CAD build for the part. Positions are in the model's coordinates, mm. A direction names the side the tool comes from. Round coordinates to 2 decimals unless told otherwise and drop trailing zeros. Loops run counter-clockwise (first coordinate to the right, second up) from the corner with the lowest first, then second, coordinate; pieces in that order, holes last.
from build123d import *

# Parameters (mm, degrees)
CUT_EXTRUDE_1_DEPTH = 4
CUT_EXTRUDE_2_DEPTH = 5


with BuildPart() as part:
    # 草图1 → 旋转1 (revolve)
    with BuildSketch(Plane(origin=(0, 0, 0), x_dir=(1, 0, 0), z_dir=(0, 1, 0)), mode=Mode.PRIVATE) as revolve_1_sk:
        Polygon((-128.123292873, 0), (-128.123292873, 15.5), (-126.123292873, 17.5), (-96.123292873, 17.5), (-96.123292873, 21), (-88.123292873, 21), (-88.123292873, 19), (-36.123292873, 19), (-36.123292873, 17.5), (5.876707127, 17.5), (5.876707127, 15), (48.876707127, 15), (48.876707127, 12.5), (106.876707127, 12.5), (108.876707127, 10.5), (108.876707127, 0), align=None)
    revolve(revolve_1_sk.sketch.rotate(Axis((-128.123292873, 0, 0), (1, 0, 0)), 180), axis=Axis((-128.123292873, 0, 0), (1, 0, 0)))

    # 草图2 → 切除-拉伸1 (cut)
    with BuildSketch(Plane(origin=(0, 0, -12.5), x_dir=(-1, 0, 0), z_dir=(0, 0, -1))):
        with BuildLine():
            Line((-101.876707127, 4), (-53.876707127, 4))
            ThreePointArc((-53.876707127, 4), (-49.876707127, 0), (-53.876707127, -4))
            Line((-53.876707127, -4), (-101.876707127, -4))
            ThreePointArc((-101.876707127, -4), (-105.876707127, 0), (-101.876707127, 4))
        make_face()
    extrude(amount=-CUT_EXTRUDE_1_DEPTH, mode=Mode.SUBTRACT)

    # 草图3 → 切除-拉伸2 (cut)
    with BuildSketch(Plane(origin=(0, 0, -19), x_dir=(-1, 0, 0), z_dir=(0, 0, -1))):
        with BuildLine():
            Line((44.123292873, 5), (79.123292873, 5))
            ThreePointArc((79.123292873, 5), (84.123292873, 0), (79.123292873, -5))
            Line((79.123292873, -5), (44.123292873, -5))
            ThreePointArc((44.123292873, -5), (39.123292873, 0), (44.123292873, 5))
        make_face()
    extrude(amount=-CUT_EXTRUDE_2_DEPTH, mode=Mode.SUBTRACT)


solid = part.part
Item 1: 3-axis set-ups, long thin cutter, end or side, ignore diameter. For faces 1 (the cylindrical face through (-39.125, -0.11, -16.536)), 2 (the flat face through (-96.123, -16, 8)), 3 (the cylindrical face through (78.283, -3.755, 11.923)), 4 (the cylindrical face through (-92.07, -6.31, 20.03)): which of +Z, -Z, +X, -X, +Y, -Y reach the whole face in a straight line?
Verdict:
face 1: -Z
face 2: -X
face 3: +X
face 4: +X, -X
Item 2: Cut at C-C (x = -110.5). List the corners of the cut face in (y, z).
Verdict:
outline: circle Ø35 at (0, 0)
Item 3: Wall check: L1, parallel to X at y = 13.5, z = -1.5; L2, parallel to Y at x = -83.5, z = -16.5; L3, parallel to X at y = 15, z = 10. Give the ranges that are in metal, low to high.
Verdict:
L1: x = -128.12 to 48.88
L2: y = -9.42 to -2.42, 2.42 to 9.42
L3: x = -96.12 to -36.12
Item 4: Cut at B-B (x = 18.5). List the corners of the cut face in (y, z).
Verdict:
outline: circle Ø30 at (0, 0)
Item 5: Flat gauge pins, fed straight in: P1, Ø5, axis at x = -65.5, y = 2, coming from the -Z side; P2, Ø12, axis at x = -61, y = -16, coming from the -Z side; P3, Ø1.5, axis at x = -8, z = 14.5, coming from the +Y side. Where does each tip first touch, or does it go through?
Verdict:
P1: stops at z = -14
P2: stops at z = -16.16
P3: stops at y = 10.83
Item 6: Cut at A-A (z = 0). List the corners of the cut face in (x, y), plus the area to 3 significant figures.
Verdict:
outline: (-128.12, -15.5) - (-126.12, -17.5) - (-96.12, -17.5) - (-96.12, -21) - (-88.12, -21) - (-88.12, -19) - (-36.12, -19) - (-36.12, -17.5) - (5.88, -17.5) - (5.88, -15) - (48.88, -15) - (48.88, -12.5) - (106.88, -12.5) - (108.88, -10.5) - (108.88, 10.5) - (106.88, 12.5) - (48.88, 12.5) - (48.88, 15) - (5.88, 15) - (5.88, 17.5) - (-36.12, 17.5) - (-36.12, 19) - (-88.12, 19) - (-88.12, 21) - (-96.12, 21) - (-96.12, 17.5) - (-126.12, 17.5) - (-128.12, 15.5) - close
area: 7,680 mm2
Item 7: Mould opens along Y. For faces 5 (the cylindrical face through (-61.76, 7.28, 17.55)), 6 (the flat face through (-62, 0, -14)), 7 (the flat face through (-61, 5, -16)), 8 (the flat face through (48.877, -12.3, -3.4)) say: released by +Y, released by -Y, zero draft, split by the parting line, or undercut.
Verdict:
face 5: split by the parting line
face 6: undercut
face 7: undercut
face 8: zero draft
